from build123d import *

# Parameters (mm, degrees)
SKETCH_1_W      = 20
SKETCH_1_H      = 20.4
EXTRUDE_1_DEPTH = 2


with BuildPart() as part:
    # 草图1 → 凸台-拉伸1 (new body)
    with BuildSketch(Plane.XY):
        with Locations((-8.175518001, 7.839742025)):
            Rectangle(SKETCH_1_W, SKETCH_1_H)
        with BuildLine():
            Line((-13.175518001, 13.539742025), (-3.175518001, 13.539742025))
            ThreePointArc((-3.175518001, 13.539742025), (-1.575518001, 11.939742025), (-3.175518001, 10.339742025))
            Line((-3.175518001, 10.339742025), (-13.175518001, 10.339742025))
            ThreePointArc((-13.175518001, 10.339742025), (-14.775518001, 11.939742025), (-13.175518001, 13.539742025))
        make_face(mode=Mode.SUBTRACT)
        with BuildLine():
            Line((-13.175518001, 0.139742025), (-3.175518001, 0.139742025))
            ThreePointArc((-3.175518001, 0.139742025), (-1.575518001, 1.739742025), (-3.175518001, 3.339742025))
            Line((-3.175518001, 3.339742025), (-13.175518001, 3.339742025))
            ThreePointArc((-13.175518001, 3.339742025), (-14.775518001, 1.739742025), (-13.175518001, 0.139742025))
        make_face(mode=Mode.SUBTRACT)
    extrude(amount=EXTRUDE_1_DEPTH)


solid = part.part
Geometry check sheet. Reference: the model listing, model coordinates, mm. A direction names the side the tool comes from. Give positions to 0.01 mm unless a question says otherwise; leave off trailing zeros. Loops run counter-clockwise (first coordinate to the right, second up) from the corner with the lowest first, then second, coordinate; pieces in that order, holes last. Notation, with made-up numbers: M 77.25,58 L 104.25,58 A10 cw 104.25,74 Z; hole C -25,20.5 d1. An arc over 180 degrees is marked long. Write each question's results on one line, items separated by ' | '.
1) Release check for a two-part mould opening along X. For faces 1 (the face through (-14.775, 1.775, 0.986)), 2 (the face through (-8, 8, 2)), 3 (the face through (-18.176, 8, 1)) record: +X half, -X half, draft (parallel to the pull), parting line (faces both ways), or undercut.
Answers follow:
face 1: undercut | face 2: draft | face 3: -X half
2) Section check D-D, the plane x = -13.5. Record the boundary of the cut face in (y, z).
Answers follow:
outline: M -2.36,0 L 0.17,0 L 0.17,2 L -2.36,2 Z; M 3.31,0 L 10.37,0 L 10.37,2 L 3.31,2 Z; M 13.51,0 L 18.04,0 L 18.04,2 L 13.51,2 Z
3) Thickness scan on line 1 (Y direction, x = -10.75, z = 1.65); line 2 (Y direction, x = -14, z = 0.4); line 3 (X direction, y = 13, z = 1.9). Record the ranges inside material, lowest first.
Answers follow:
line 1: -2.36 to 0.14, 3.34 to 10.34, 13.54 to 18.04 | line 2: -2.36 to 0.37, 3.11 to 10.57, 13.31 to 18.04 | line 3: -18.18 to -14.37, -1.98 to 1.82
4) Section check A-A, the plane x = -5.75. Record the boundary of the cut face in (y, z), plus the area to 3 significant figures.
Answers follow:
outline: M -2.36,0 L 0.14,0 L 0.14,2 L -2.36,2 Z; M 3.34,0 L 10.34,0 L 10.34,2 L 3.34,2 Z; M 13.54,0 L 18.04,0 L 18.04,2 L 13.54,2 Z | area: 28.0 mm2
5) Section check B-B, the plane z = 0.85. Record the boundary of the cut face in (x, y).
Answers follow:
outline: M -18.18,-2.36 L 1.82,-2.36 L 1.82,18.04 L -18.18,18.04 Z; hole M -13.18,0.14 L -3.18,0.14 A1.6 ccw -3.18,3.34 L -13.18,3.34 A1.6 ccw Z; hole M -13.18,10.34 L -3.18,10.34 A1.6 ccw -3.18,13.54 L -13.18,13.54 A1.6 ccw Z
6) Tool access check on faces 4 (the face through (-8, -2.36, 1)), 5 (the face through (-8, 10.34, 1)). Record the directions out of +Z, -Z, +X, -X, +Y, -Y that give a thin tool (end or side, any length) a straight path to the whole face; none if there is none.
Answers follow:
face 4: +Z, -Z, +X, -X, -Y | face 5: +Z, -Z
7) Gauge pin test, flat end, axial feed: pin 1 (1 mm diameter, centred on x = -7, y = 12, fed in from -Z). Record the tip position at first contact, or that the pin passes through.
Answers follow:
pin 1: through
8) Section check C-C, the plane y = 1. Record the boundary of the cut face in (x, z).
Answers follow:
outline: M -18.18,0 L -14.59,0 L -14.59,2 L -18.18,2 Z; M -1.76,0 L 1.82,0 L 1.82,2 L -1.76,2 Z
